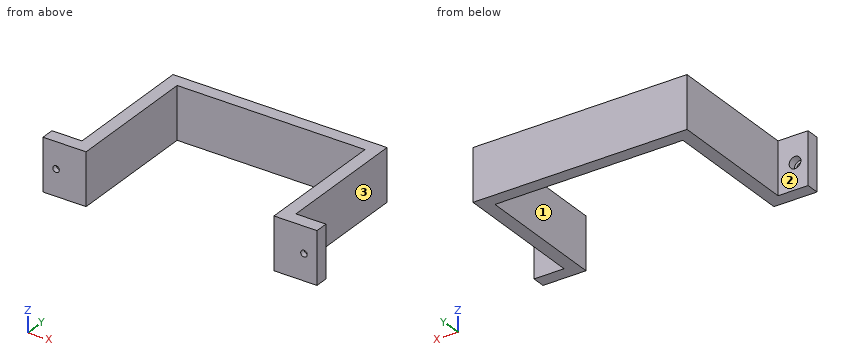
Autodesk Inventor part; units mm, degrees
ref_plane "YZ Plane" through (0, 0, 0) normal (1, 0, 0) x (0, 1, 0)
ref_plane "XZ Plane" through (0, 0, 0) normal (0, 1, 0) x (-1, 0, 0)
ref_plane "XY Plane" through (0, 0, 0) normal (0, 0, 1) x (1, 0, 0)
sketch "Sketch1" plane through (0, 0, 0) normal (0, 0, 1) x (1, 0, 0)
  line L0 (-52.5, 5) -> (-41, 5)
  line L1 (-41, 5) -> (-41, 56)
  line L2 (-41, 56) -> (41, 56)
  line L3 (41, 56) -> (41, 5)
  line L4 (41, 5) -> (52.5, 5)
  line L5 (-36, 0) -> (-36, 51)
  line L6 (-36, 51) -> (36, 51)
  line L7 (36, 51) -> (36, 0)
  line L8 (0, 0) -> (0, -25.7238) construction
  line L9 (52.5, 0) -> (52.5, 5)
  line L10 (-52.5, 0) -> (-52.5, 5)
  line L11 (-52.5, 0) -> (-36, 0)
  line L12 (36, 0) -> (52.5, 0)
  dimension "d1" = 5
  dimension "d2" = 5
  dimension "d3" = 5
  dimension "d5" = 72
  dimension "d6" = 51
  dimension "d7" = 16.5
  dimension "d8" = 5
extrude "Extrusion1" add sketch "Sketch1" along normal mid plane 20
sketch "Sketch2" plane through (-52.5, 0, 10) normal (0, -1, 0) x (1, 0, 0)
  circle A0 centre (5, -10) radius 1.25
  circle A1 centre (100, -10) radius 1.25
  line L0 (52.5, -10) -> (52.5, 0) construction
  line L1 (16.5, 0) -> (88.5, 0) construction
  circle A2 centre (5, -10) radius 2.25
  circle A3 centre (100, -10) radius 2.25
  dimension "d11" = 2.5
  dimension "d12" = 95
  dimension "d15" = 4.5
extrude "Extrusion2" cut sketch "Sketch2" against normal through all contours A0 | A1
extrude "Extrusion3" cut sketch "Sketch2" along normal blind 3 from surface at -5
equation "\"d1\" = d8"
equation "\"d2\" = d8"
equation "\"d3\" = d8"
properties part number "battery_fix"
The model under review builds one solid part; all positions refer to its coordinate system, in mm. Face numbers are marked on the shaded views. A direction names the side the tool comes from. Round coordinates to 2 decimals unless told otherwise and drop trailing zeros. Loops run counter-clockwise (first coordinate to the right, second up) from the corner with the lowest first, then second, coordinate; pieces in that order, holes last. Notation, with made-up numbers: (-16, 85.5) -> (-7, 85.5) arc R14 cw to (-7, 111.5) -> close; hole circle Ø4 at (-11, -1.5). An arc over 180 degrees is marked (long way). Answer as a JSON object with one key per item and string values. Group by question number.
1) For pin 1 Ø7 at (x, z) = (47.5, 0) entering from +Y; pin 2 Ø5 at (y, z) = (45.5, -2) entering from -X; pin 3 Ø2 at (x, z) = (-48, -0.5) entering from +Y; pin 4 Ø2 at (x, z) = (47.5, 0) entering from +Y, all flat-tipped, find the tip position at first contact; note any pin that passes through.
2) We need section B-B on y = 32. Write out the cut boundary in (x, z), then the cut area to 3 significant figures.
3) We need section D-D on z = 7.5. Write out the cut boundary in (x, y).
4) For the marked faces 1, 2 and 3, list the 3-axis set-ups (+Z, -Z, +X, -X, +Y, -Y) from which the entire face can be reached by the end or side of a thin tool; tool diameter is ignored.
5) For line 1 (Z direction, x = -47.5, y = 0.6); line 2 (Z direction, x = -47.5, y = 3.6); line 3 (X direction, y = 25, z = -8.75), list the stretches that pass through material, from the lowest coordinate up. Write a range as [from, to].
6) We need section C-C on z = 0. Write out the cut boundary in (x, y).
7) We need section A-A on x = -47.5. Write out the cut boundary in (y, z), then the cut area to 3 significant figures.
Result set:
{
 "1": {"pin 1": "y = 5", "pin 2": "x = -41", "pin 3": "y = 2", "pin 4": "through"},
 "2": {"outline": "(-41, -10) -> (-36, -10) -> (-36, 10) -> (-41, 10) -> close; (36, -10) -> (41, -10) -> (41, 10) -> (36, 10) -> close", "area": "200 mm²"},
 "3": {"outline": "(-52.5, 0) -> (-36, 0) -> (-36, 51) -> (36, 51) -> (36, 0) -> (52.5, 0) -> (52.5, 5) -> (41, 5) -> (41, 56) -> (-41, 56) -> (-41, 5) -> (-52.5, 5) -> close"},
 "4": {"face 1": "+Z, -Z, -Y", "face 2": "+Z, -Z, -X, +Y", "face 3": "+Z, -Z, +X, +Y"},
 "5": {"line 1": "[-10, -1.25], [1.25, 10]", "line 2": "[-10, -2.25], [2.25, 10]", "line 3": "[-41, -36], [36, 41]"},
 "6": {"outline": "(-52.5, 0) -> (-48.75, 0) -> (-48.75, 2) -> (-49.75, 2) -> (-49.75, 5) -> (-52.5, 5) -> close; (-46.25, 0) -> (-36, 0) -> (-36, 51) -> (36, 51) -> (36, 0) -> (46.25, 0) -> (46.25, 2) -> (45.25, 2) -> (45.25, 5) -> (41, 5) -> (41, 56) -> (-41, 56) -> (-41, 5) -> (-45.25, 5) -> (-45.25, 2) -> (-46.25, 2) -> close; (48.75, 0) -> (52.5, 0) -> (52.5, 5) -> (49.75, 5) -> (49.75, 2) -> (48.75, 2) -> close"},
 "7": {"outline": "(0, -10) -> (5, -10) -> (5, -2.25) -> (2, -2.25) -> (2, -1.25) -> (0, -1.25) -> close; (0, 1.25) -> (2, 1.25) -> (2, 2.25) -> (5, 2.25) -> (5, 10) -> (0, 10) -> close", "area": "81.5 mm²"}
}
